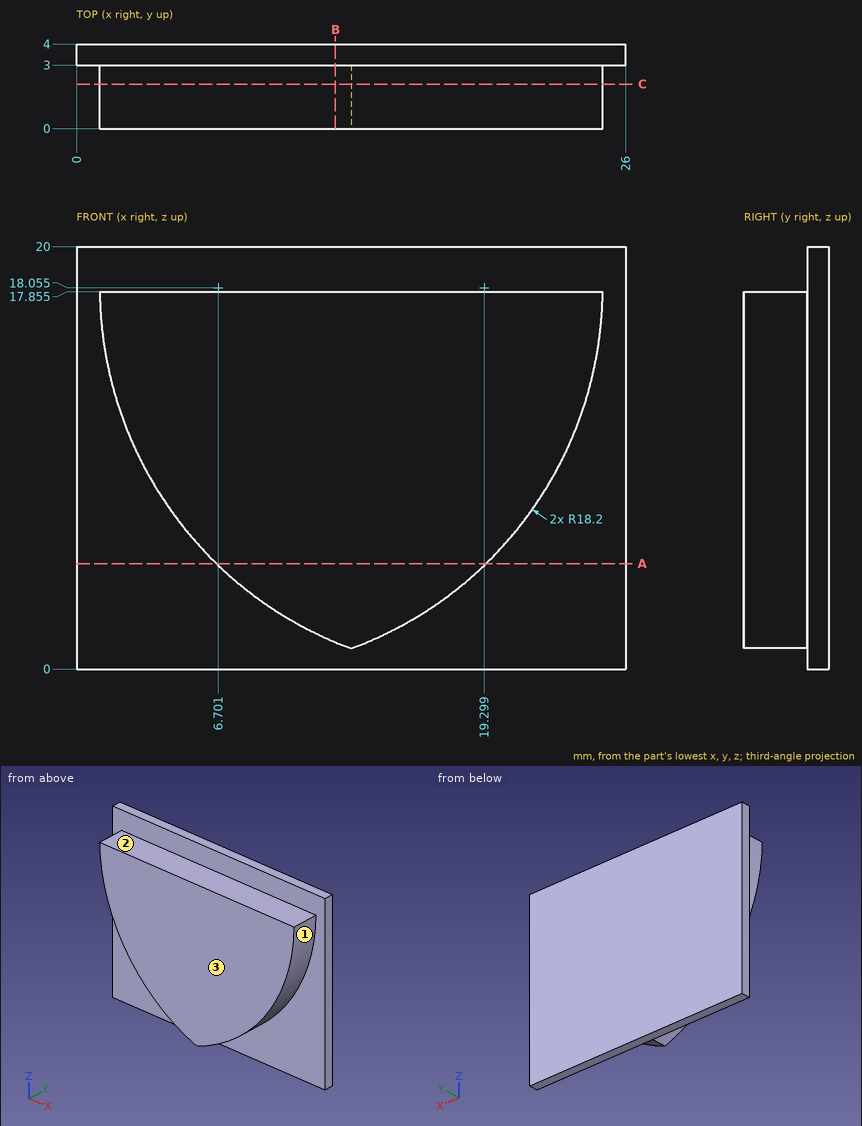
Study the drawing (mm; zero at the part's minimum x, y, z) and answer. A direction names the side the tool comes from. Give positions to 0.01 mm unless a question says otherwise; leave off trailing zeros. Order: outer loops, then holes, each group sorted by start corner. A loop starts at its lowest first (then second) coordinate and runs counter-clockwise, first axis right, second up. Notation, with made-up numbers: (67.25, 64.25) -> (89.25, 64.25) arc R13 ccw to (89.25, 86.25) -> close; hole circle Ø2 at (33, 23). An arc over 180 degrees is marked (long way). Write item = value, one per line.
1. A cutting plane is placed at C-C, the plane y = 2.1. Write down the section's boundary in (x, z) (3 decimals).
Numbers:
outline = (1.1, 17.855) arc R18.2 ccw to (13, 0.98) arc R18.2 ccw to (24.9, 17.855) -> close
2. Given pin 1 (2 mm diameter, centred on x = 4.5, y = 1.5, fed in from -Z); pin 2 (1 mm diameter, centred on x = 5.5, y = 2, fed in from +Z) (3 decimals), each flat-ended and moving along its own axis, determine where each tip first touches the part or whether it passes through.
Numbers:
pin_1 = 6.19
pin_2 = 17.855
3. A cutting plane is placed at B-B, the plane x = 12.25. Write down the section's boundary in (y, z) (1 decimal).
Numbers:
outline = (0, 1.3) -> (3, 1.3) -> (3, 0) -> (4, 0) -> (4, 20) -> (3, 20) -> (3, 17.9) -> (0, 17.9) -> close
4. Straight lines are drawn through the part: line 1 along Y through (x, z) = (20.5, 5.75); line 2 along X through (y, z) = (2.85, 8); line 3 along X through (y, z) = (1.6, 4). For each, find the intervals that lie inside material, in ascending order.
Numbers:
line_1 = 3 to 4
line_2 = 4.13 to 21.87
line_3 = 7.74 to 18.26
5. A cutting plane is placed at A-A, the plane z = 5. Write down the section's boundary in (x, y), and give its area (3 significant figures).
Numbers:
outline = (0, 3) -> (6.62, 3) -> (6.62, 0) -> (19.38, 0) -> (19.38, 3) -> (26, 3) -> (26, 4) -> (0, 4) -> close
area = 64.3 mm²
6. For the marked faces 1, 2 and 3, determine the directions among +Z, -Z, +X, -X, +Y, -Y from which every point of the face is accessible in a straight line to the end or side of a thin tool.
Numbers:
face_1 = -Z, +X, -Y
face_2 = +Z, +X, -X, -Y
face_3 = +Z, -Z, +X, -X, -Y
